Here's how the part is built. I have some questions about the finished solid (model axes, mm). Give positions to 0.01 mm unless a question says otherwise; leave off trailing zeros. Loops run counter-clockwise (first coordinate to the right, second up) from the corner with the lowest first, then second, coordinate; pieces in that order, holes last.
Q1. If we section it at B-B (z = 7.5): Please give me the cut outline in (x, y).
Q2. I need wall thicknesses on line 1 (X direction, y = -8, z = 14.25); line 2 (Z direction, x = 26.5, y = -6); line 3 (X direction, y = -13.75, z = 3). Which ranges of each line are inside material? Lowest first, please.
Q3. If we section it at C-C (z = 10.5): Please give me the cut outline in (x, y), plus the area to 3 significant figures.
Q4. If we section it at D-D (y = -6.5): Please give me the cut outline in (x, z).
Q5. We'd pull the mould along X, two halves only. Please class faces 1 (the face through (27.814, -12.381, 6.036)), 2 (the face through (0, -21, 7)), 3 (the face through (-28.05, -12.62, 3.08)): +X half, -X half, draft (parallel to the pull), parting line (faces both ways), or undercut.
Q6. Will these pins go through, and if not, where does the flat tip stop? P1, Ø0.8, axis at x = -21, z = 9.5, coming from the +Y side; P2, Ø6, axis at x = -11, z = 4.5, coming from the +Y side; P3, Ø5, axis at y = -16, z = 2, coming from the -X side.
Q7. If we section it at A-A (y = -16.75): Please give me the cut outline in (x, z).
from build123d import *

# Parameters (mm, degrees)
BOSS_EXTRUDE1_DEPTH = 15
CHAMFER1_SIZE       = 2.5
SKETCH2_R           = 1.5
CUT_EXTRUDE1_DEPTH  = 40.667340007
SKETCH3_W           = 0.942684348
SKETCH3_H           = 15
CUT_EXTRUDE2_DEPTH  = 1
CUT_EXTRUDE3_DEPTH  = 25


with BuildPart() as part:
    # Sketch1 → Boss-Extrude1 (new body)
    with BuildSketch(Plane.XY):
        with BuildLine():
            Line((-17.549928775, -4), (-32.549928775, -4))
            Line((-32.549928775, -4), (-32.549928775, -21))
            Line((-32.549928775, -21), (32.549928775, -21))
            Line((32.549928775, -21), (32.549928775, -4))
            Line((32.549928775, -4), (17.549928775, -4))
            ThreePointArc((17.549928775, -4), (0, -18), (-17.549928775, -4))
        make_face()
    extrude(amount=BOSS_EXTRUDE1_DEPTH)

    # Chamfer1
    chamfer1_edges = [part.edges().sort_by_distance(p)[0] for p in [
        (-32.549928775, -12.5, 15),
        (32.549928775, -12.5, 15),
        (32.549928775, -12.5, 0),
    ]]
    chamfer(chamfer1_edges, length=CHAMFER1_SIZE)

    # Sketch2 → Cut-Extrude1 (cut, through all)
    with BuildSketch(Plane(origin=(0, -4, 0), x_dir=(1, 0, 0), z_dir=(0, 1, 0))):
        with Locations(Location((27.488644481, -7.5, 0), (0, 0, 180))):
            Circle(SKETCH2_R)
        with Locations((-27.488644481, -7.5)):
            Circle(SKETCH2_R)
    extrude(amount=-CUT_EXTRUDE1_DEPTH, mode=Mode.SUBTRACT)

    # Sketch3 → Cut-Extrude2 (cut)
    with BuildSketch(Plane(origin=(0, -4, 0), x_dir=(1, 0, 0), z_dir=(0, 1, 0))):
        with Locations((-21.008394031, -7.5)):
            Rectangle(SKETCH3_W, SKETCH3_H)
    cut_extrude2 = extrude(amount=-CUT_EXTRUDE2_DEPTH, mode=Mode.SUBTRACT)

    # Mirror1: Cut-Extrude2 across plane
    add(cut_extrude2.mirror(Plane(origin=(0, 0, 0), x_dir=(0, 0, 1), z_dir=(1, 0, 0))), mode=Mode.SUBTRACT)

    # Sketch4 → Cut-Extrude3 (cut)
    with BuildSketch(Plane.XZ.offset(21)):
        Polygon((-23.68309692, 0), (-32.549928775, 6.25), (-32.549928775, 0), align=None)
    extrude(amount=-CUT_EXTRUDE3_DEPTH, mode=Mode.SUBTRACT)


solid = part.part
Check sheet entries:
1. outline: (-32.55, -21) - (-28.99, -21) - (-28.99, -4) - (-32.55, -4) - close; (-25.99, -21) - (25.99, -21) - (25.99, -4) - (21.48, -4) - (21.48, -5) - (20.54, -5) - (20.54, -4) - (17.55, -4) arc R18 cw to (-17.55, -4) - (-20.54, -4) - (-20.54, -5) - (-21.48, -5) - (-21.48, -4) - (-25.99, -4) - close; (28.99, -21) - (32.55, -21) - (32.55, -4) - (28.99, -4) - close
2. line 1: x = -30.8 to -16.12, 16.12 to 30.8
2. line 2: z = 0 to 6.37, 8.63 to 15
2. line 3: x = -27.94 to -11.62, 11.62 to 32.55
3. outline: (-32.55, -21) - (32.55, -21) - (32.55, -4) - (21.48, -4) - (21.48, -5) - (20.54, -5) - (20.54, -4) - (17.55, -4) arc R18 cw to (-17.55, -4) - (-20.54, -4) - (-20.54, -5) - (-21.48, -5) - (-21.48, -4) - (-32.55, -4) - close
3. area: 739 mm2
4. outline: (-32.55, 6.25) - (-23.68, 0) - (-16.79, 0) - (-16.79, 15) - (-30.05, 15) - (-32.55, 12.5) - close; (16.79, 0) - (30.05, 0) - (32.55, 2.5) - (32.55, 12.5) - (30.05, 15) - (16.79, 15) - close; hole circle Ø3 at (-27.49, 7.5); hole circle Ø3 at (27.49, 7.5)
5. face 1: undercut
5. face 2: draft
5. face 3: -X half
6. P1: stops at y = -5
6. P2: stops at y = -11.31
6. P3: stops at x = -30.07
7. outline: (-32.55, 6.25) - (-23.68, 0) - (-6.59, 0) - (-6.59, 15) - (-30.05, 15) - (-32.55, 12.5) - close; (6.59, 0) - (30.05, 0) - (32.55, 2.5) - (32.55, 12.5) - (30.05, 15) - (6.59, 15) - close; hole circle Ø3 at (-27.49, 7.5); hole circle Ø3 at (27.49, 7.5)
